The figure shows three views and two pictorial views of one solid part (mm, origin at its lowest corner). Answer the questions. A direction names the side the tool comes from. Give positions to 0.01 mm unless a question says otherwise; leave off trailing zeros. Write each loop counter-clockwise with the first axis right and the second up, starting at its lowest first coordinate (ties: lowest second). Pieces come first, ordered by that corner, then holes. Notation, with made-up numbers: (0, 44.5) - (16, 44.5) arc R28 ccw to (16, 68.5) - close; hole circle Ø4 at (-17, 89). An arc over 180 degrees is marked (long way). Use a Markdown table: item, result. Add a question column.
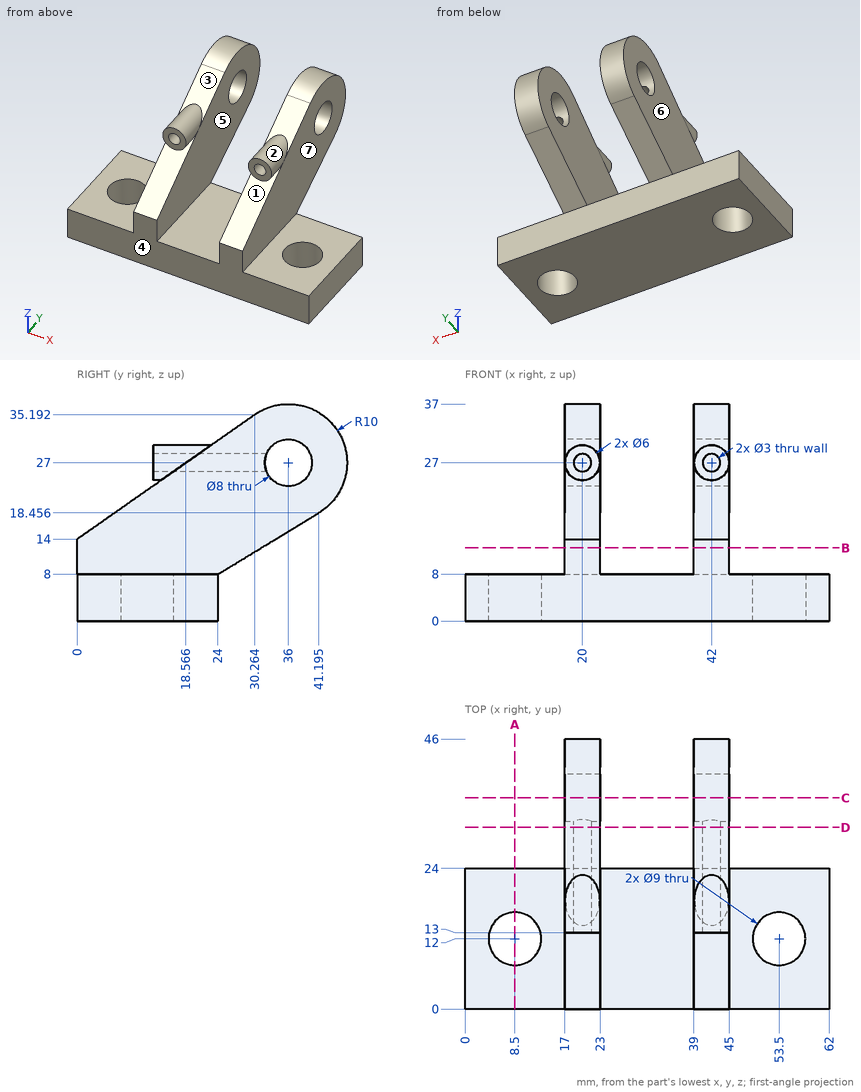
1. Consider L1, parallel to X at y = 18.5, z = 27; L2, parallel to Y at x = 53.5, z = 4.5; L3, parallel to X at y = 29.5, z = 24. Determine where each line is inside the solid, lowest interval first. Write a range as [from, to].
2. Which of the six approach directions +Z, -Z, +X, -X, +Y, -Y give full straight-line access (tool end or side, diameter ignored) to the marked faces 5, 6 and 7?
3. The part is cut by section D-D (y = 31). Give the vertices of the cut face in (x, z), and give its area (3 significant figures).
4. The part is cut by section A-A (x = 8.5). Give the vertices of the cut face in (y, z).
5. The part is cut by section B-B (z = 12.5). Give the vertices of the cut face in (x, y).
6. The part is cut by section C-C (y = 36). Give the vertices of the cut face in (x, z).
7. For a pull along Z with two mould halves and no side action, classify the marked faces 1, 2, 3 and 4 as released by +Z, released by -Z, zero draft, split by the parting line, or undercut.
8. Given P1, Ø9, axis at x = 16, z = 4, coming from the +Y side (1 decimal); P2, Ø11.5, axis at x = 8.5, y = 12, coming from the +Z side; P3, Ø5, axis at x = 45, z = 29, coming from the -Y side, each flat-ended and moving along its own axis, determine where each tip first touches the part or whether it passes through.
Check values:
| question | item | result |
|---|---|---|
| 1 | L1 | x = [17, 18.5], [21.5, 23], [39, 40.5], [43.5, 45] |
| 1 | L2 | y = [0, 7.5], [16.5, 24] |
| 1 | L3 | x = [17, 23], [39, 45] |
| 2 | face 5 | +Z, +Y, -Y |
| 2 | face 6 | +Z, -X, +Y, -Y |
| 2 | face 7 | +Z, +X, +Y, -Y |
| 3 | outline | (17, 12.26) - (23, 12.26) - (23, 35.66) - (17, 35.66) - close; (39, 12.26) - (45, 12.26) - (45, 35.66) - (39, 35.66) - close; hole circle Ø3 at (20, 27); hole circle Ø3 at (42, 27) |
| 3 | area | 267 mm2 |
| 4 | outline | (0, 0) - (7.5, 0) - (7.5, 8) - (0, 8) - close; (16.5, 0) - (24, 0) - (24, 8) - (16.5, 8) - close |
| 5 | outline | (17, 0) - (23, 0) - (23, 31.4) - (17, 31.4) - close; (39, 0) - (45, 0) - (45, 31.4) - (39, 31.4) - close |
| 6 | outline | (17, 15.3) - (23, 15.3) - (23, 23) - (17, 23) - close; (17, 31) - (23, 31) - (23, 37) - (17, 37) - close; (39, 15.3) - (45, 15.3) - (45, 23) - (39, 23) - close; (39, 31) - (45, 31) - (45, 37) - (39, 37) - close |
| 7 | face 1 | undercut |
| 7 | face 2 | undercut |
| 7 | face 3 | released by +Z |
| 7 | face 4 | zero draft |
| 8 | P1 | stops at y = 24.6 |
| 8 | P2 | stops at z = 8 |
| 8 | P3 | stops at y = 13 |
